Read the model definition and answer for the solid it produces. Units are mm, in the model's axes. A direction names the side the tool comes from. Give positions to 0.01 mm unless a question says otherwise; leave off trailing zeros. Write each loop counter-clockwise with the first axis right and the second up, starting at its lowest first coordinate (ties: lowest second). Pieces come first, ordered by that corner, then holes. Notation, with made-up numbers: (-36.75, 58.5) - (11.25, 58.5) arc R24 ccw to (11.25, 84.5) - close; hole circle Ø1 at (22, 52). An arc over 180 degrees is marked (long way). Answer as CSV lines item,"result".
```python
from build123d import *

# Parameters (mm, degrees)
SZKIC1_W                    = 7.6
SZKIC1_H                    = 5.6
DODANIE_WYCI_GNI_CIE1_DEPTH = 5
DODANIE_WYCI_GNI_CIE2_DEPTH = 5
SZKIC3_W                    = 3.6
SZKIC3_H                    = 7
DODANIE_WYCI_GNI_CIE3_DEPTH = 5
SZKIC4_R                    = 2.3
DODANIE_WYCI_GNI_CIE4_DEPTH = 5
SFAZOWANIE1_SIZE            = 3
DODANIE_WYCI_GNI_CIE5_DEPTH = 7.6


with BuildPart() as part:
    # Szkic1 → Dodanie-wyciągnięcie1 (new body)
    with BuildSketch(Plane.XY):
        Rectangle(SZKIC1_W, SZKIC1_H)
    extrude(amount=DODANIE_WYCI_GNI_CIE1_DEPTH)

    # Szkic2 → Dodanie-wyciągnięcie2 (add)
    with BuildSketch(Plane.XY.offset(5)):
        with BuildLine():
            Line((-6.955089184, -1.3), (-6.955089184, 1.3))
            Line((-6.955089184, 1.3), (-5.602633404, 1.3))
            ThreePointArc((-5.602633404, 1.3), (-9.8, 0), (-5.602633404, -1.3))
            Line((-5.602633404, -1.3), (-6.955089184, -1.3))
        make_face()
        with BuildLine():
            Line((-5.602633404, 1.3), (-6.955089184, 1.3))
            Line((-6.955089184, 1.3), (-6.955089184, -1.3))
            Line((-6.955089184, -1.3), (-5.602633404, -1.3))
            ThreePointArc((-5.602633404, -1.3), (-5.302962999, -0.680461913), (-5.2, 0))
            ThreePointArc((-5.2, 0), (-5.302962999, 0.680461913), (-5.602633404, 1.3))
        make_face()
        with BuildLine():
            Line((-3.8, 1.3), (-5.602633404, 1.3))
            ThreePointArc((-5.602633404, 1.3), (-5.302962999, 0.680461913), (-5.2, 0))
            ThreePointArc((-5.2, 0), (-5.302962999, -0.680461913), (-5.602633404, -1.3))
            Line((-5.602633404, -1.3), (-3.8, -1.3))
            Line((-3.8, -1.3), (-3.8, 1.3))
        make_face()
    extrude(amount=-DODANIE_WYCI_GNI_CIE2_DEPTH)

    # Szkic3 → Dodanie-wyciągnięcie3 (add)
    with BuildSketch(Plane.XY.offset(5)):
        with Locations((-2, -6.3)):
            Rectangle(SZKIC3_W, SZKIC3_H)
    extrude(amount=-DODANIE_WYCI_GNI_CIE3_DEPTH)

    # Szkic4 → Dodanie-wyciągnięcie4 (add)
    with BuildSketch(Plane(origin=(0, 0, 0), x_dir=(-1, 0, 0), z_dir=(0, 0, -1))):
        with Locations(Location((7.5, 0, 0), (0, 0, 145.58261129))):
            Circle(SZKIC4_R)
    extrude(amount=DODANIE_WYCI_GNI_CIE4_DEPTH)

    # Sfazowanie1
    sfazowanie1_edges = [part.edges().sort_by_distance(p)[0] for p in [
        (-2, -9.8, 5),
    ]]
    chamfer(sfazowanie1_edges, length=SFAZOWANIE1_SIZE)

    # Szkic5 → Dodanie-wyciągnięcie5 (add)
    with BuildSketch(Plane(origin=(3.8, 0, 0), x_dir=(0, 0, -1), z_dir=(1, 0, 0))):
        Polygon((-5, 2.8), (-8.5, 2.8), (-8.5, 1.8), (-5, -2.8), align=None)
    extrude(amount=-DODANIE_WYCI_GNI_CIE5_DEPTH)


solid = part.part
```
(1) A cutting plane is placed at B-B (x = 2.5). Write down the section's boundary in (y, z), and give its area (4 significant figures).
Worked out:
outline,"(-2.8, 0) - (2.8, 0) - (2.8, 8.5) - (1.8, 8.5) - (-2.8, 5) - close"
area,"39.55 mm^2"
(2) Each of these flat-tipped pins is pushed along its axis until it touches: P1, Ø4, axis at y = -7.5, z = 3.5, coming from the +X side; P2, Ø1.4, axis at x = -7, y = -1, coming from the +Z side; P3, Ø7.5, axis at x = 1.5, y = -1.5, coming from the -Z side. Where does it stop, or does it pass through?
Worked out:
P1,"stops at x = -0.2"
P2,"stops at z = 5"
P3,"stops at z = 0"
(3) Find the intervals of material crossed by L1, parallel to X at y = 0.5, z = 6; L2, parallel to X at y = -7.5, z = 1.5; L3, parallel to Y at x = 0.25, z = 4.25, in increasing order.
Worked out:
L1,"x = -3.8 to 3.8"
L2,"x = -3.8 to -0.2"
L3,"y = -2.8 to 2.8"
(4) A cutting plane is placed at D-D (x = -7.5). Write down the section's boundary in (y, z), and give its area (3 significant figures).
Worked out:
outline,"(-2.3, -5) - (2.3, -5) - (2.3, 5) - (-2.3, 5) - close"
area,"46.0 mm^2"
(5) A cutting plane is placed at C-C (y = 0). Write down the section's boundary in (x, z), and give its area (3 significant figures).
Worked out:
outline,"(-9.8, -5) - (-5.2, -5) - (-5.2, 0) - (3.8, 0) - (3.8, 7.13) - (-3.8, 7.13) - (-3.8, 5) - (-9.8, 5) - close"
area,"107 mm^2"
(6) The mould has two halves that part along X. Classify faces 5 (the flat face through (-2, -8.3, 3.5)), 6 (the flat face through (3.8, 0, 3)), 7 (the flat face through (-3.8, -3, 3)): +X half, -X half, draft (parallel to the pull), parting line (faces both ways), or undercut.
Worked out:
face 5,"draft"
face 6,"+X half"
face 7,"undercut"
(7) For faces 1 (the flat face through (-7, 0, 5)), 2 (the flat face through (-2, -5, 5)), 3 (the flat face through (-5, -1.3, 3)), 4 (the flat face through (2, -2.8, 2)), determine the directions among +Z, -Z, +X, -X, +Y, -Y from which every point of the face is accessible in a straight line to the end or side of a thin tool.
Worked out:
face 1,"+Z, -X, +Y, -Y"
face 2,"+Z, +X, -X, -Y"
face 3,"+Z, -Z, -Y"
face 4,"+Z, -Z, +X, -Y"
(8) A cutting plane is placed at A-A (z = 1). Write down the section's boundary in (x, y), and give its area (3 significant figures).
Worked out:
outline,"(-5.6, -1.3) - (-3.8, -1.3) - (-3.8, -9.8) - (-0.2, -9.8) - (-0.2, -2.8) - (3.8, -2.8) - (3.8, 2.8) - (-3.8, 2.8) - (-3.8, 1.3) - (-5.6, 1.3) arc R2.3 ccw (long way) to start"
area,"88.4 mm^2"
